For this review, use the dimensioned drawing (mm, ordinates from the lowest corner) and the shaded views. Round coordinates to 2 decimals unless told otherwise and drop trailing zeros. Loops run counter-clockwise (first coordinate to the right, second up) from the corner with the lowest first, then second, coordinate; pieces in that order, holes last. Notation, with made-up numbers: (61.5, 80) -> (113.5, 80) arc R26 cw to (113.5, 111) -> close; hole circle Ø9 at (25.5, 20.25). An arc over 180 degrees is marked (long way). Answer as CSV lines item,"result". Start each with the question number.
(1) To check wall thickness, follow line 1 (X direction, y = 14, z = 14.5) (3 decimals); line 2 (Y direction, x = 23.85, z = 203.2). State the ranges of each line that lie inside material, in increasing order. Write a range as from..to.
(2) Take a section at A-A, the plane y = 12.7. Write out the cut boundary in (x, z) (3 decimals).
(3) Take a section at D-D, the plane z = 158. Write out the cut boundary in (x, y) (3 decimals).
(4) Take a section at C-C, the plane z = 25.4. Write out the cut boundary in (x, y) (3 decimals), and give its area (3 significant figures).
(5) Take a section at B-B, the plane x = 15. Write out the cut boundary in (y, z) (3 decimals), and give its area (3 significant figures).
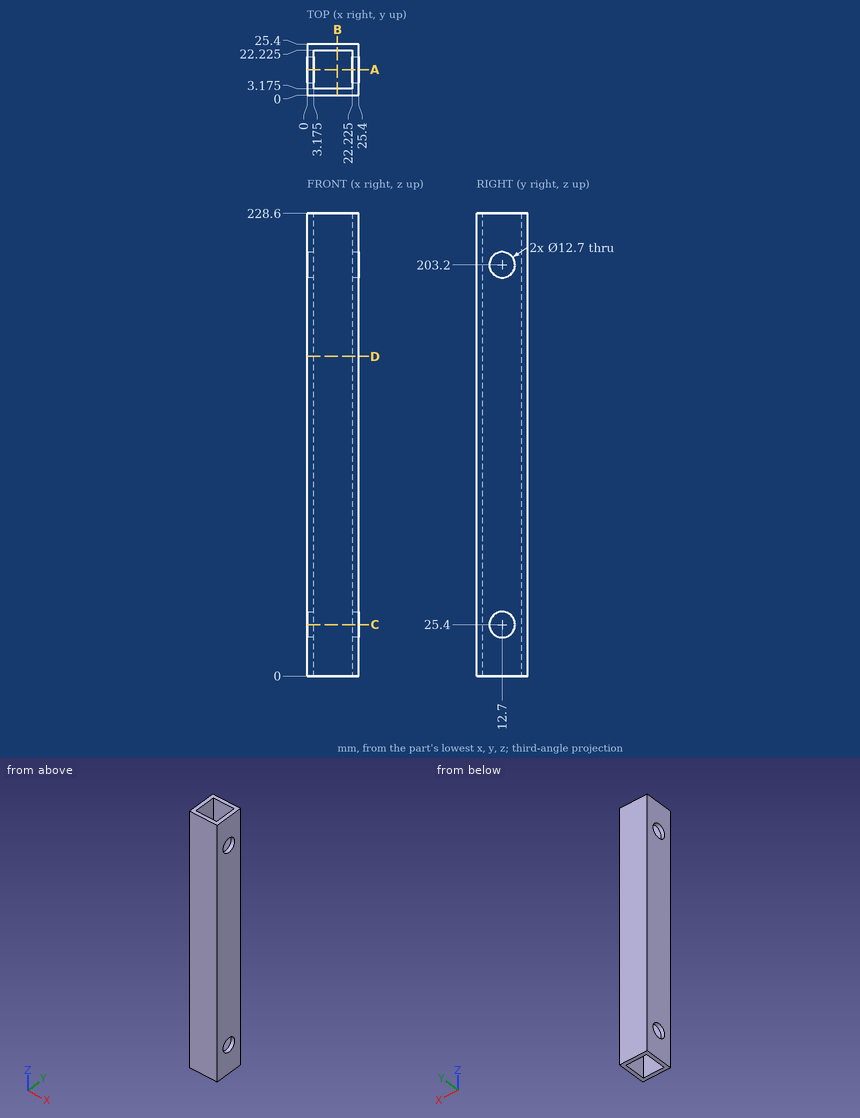
The answers:
1,line 1,"0..3.175, 22.225..25.4"
1,line 2,"0..6.35, 19.05..25.4"
2,outline,"(0, 0) -> (3.175, 0) -> (3.175, 19.05) -> (0, 19.05) -> close; (0, 31.75) -> (3.175, 31.75) -> (3.175, 196.85) -> (0, 196.85) -> close; (0, 209.55) -> (3.175, 209.55) -> (3.175, 228.6) -> (0, 228.6) -> close; (22.225, 0) -> (25.4, 0) -> (25.4, 19.05) -> (22.225, 19.05) -> close; (22.225, 31.75) -> (25.4, 31.75) -> (25.4, 196.85) -> (22.225, 196.85) -> close; (22.225, 209.55) -> (25.4, 209.55) -> (25.4, 228.6) -> (22.225, 228.6) -> close"
3,outline,"(0, 0) -> (25.4, 0) -> (25.4, 25.4) -> (0, 25.4) -> close; hole (3.175, 3.175) -> (22.225, 3.175) -> (22.225, 22.225) -> (3.175, 22.225) -> close"
4,outline,"(0, 0) -> (25.4, 0) -> (25.4, 6.35) -> (22.225, 6.35) -> (22.225, 3.175) -> (3.175, 3.175) -> (3.175, 6.35) -> (0, 6.35) -> close; (0, 19.05) -> (3.175, 19.05) -> (3.175, 22.225) -> (22.225, 22.225) -> (22.225, 19.05) -> (25.4, 19.05) -> (25.4, 25.4) -> (0, 25.4) -> close"
4,area,"202 mm²"
5,outline,"(0, 0) -> (3.175, 0) -> (3.175, 228.6) -> (0, 228.6) -> close; (22.225, 0) -> (25.4, 0) -> (25.4, 228.6) -> (22.225, 228.6) -> close"
5,area,"1,450 mm²"
